Design review of the part built by this model. Coordinates are the model's own, in mm. Face numbers are marked on the shaded views. Give positions to 0.01 mm unless a question says otherwise; leave off trailing zeros. Order: outer loops, then holes, each group sorted by start corner. A loop starts at its lowest first (then second) coordinate and runs counter-clockwise, first axis right, second up. Notation, with made-up numbers: (43.25, -39.75) -> (57.25, -39.75) arc R25 cw to (57.25, -12.75) -> close; hole circle Ø1 at (-4.5, 53). An arc over 180 degrees is marked (long way). Answer in a Markdown table with one row per item. Add a question column.
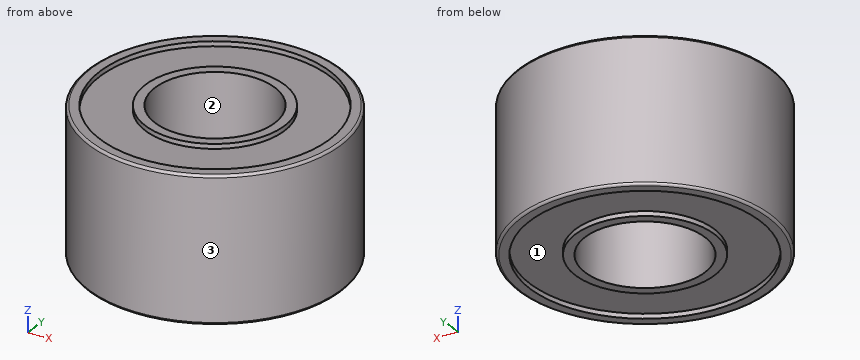
```python
from build123d import *

# Parameters (mm, degrees)
SKETCH1_R           = 10.55
SKETCH1_R_2         = 5
BOSS_EXTRUDE1_DEPTH = 6
FILLET1_R           = 0.2
SKETCH3_R           = 9.602296017
SKETCH3_R_2         = 5.812916565
CUT_EXTRUDE1_DEPTH  = 0.4


with BuildPart() as part:
    # Sketch1 → Boss-Extrude1 (new, symmetric)
    with BuildSketch(Plane.XY):
        Circle(SKETCH1_R)
        Circle(SKETCH1_R_2, mode=Mode.SUBTRACT)
    extrude(amount=BOSS_EXTRUDE1_DEPTH, both=True)

    # Fillet1
    fillet1_edges = [part.edges().sort_by_distance(p)[0] for p in [
        (-10.55, 0, -6),
        (-10.55, 0, 6),
    ]]
    fillet(fillet1_edges, radius=FILLET1_R)

    # Sketch3 → Cut-Extrude1 (cut)
    with BuildSketch(Plane.XY.offset(6)):
        Circle(SKETCH3_R)
        Circle(SKETCH3_R_2, mode=Mode.SUBTRACT)
    cut_extrude1 = extrude(amount=-CUT_EXTRUDE1_DEPTH, mode=Mode.SUBTRACT)

    # Mirror1: Cut-Extrude1 across plane
    add(cut_extrude1.mirror(Plane.XY), mode=Mode.SUBTRACT)


solid = part.part
```
1) Clearance check with flat-ended pins moving along their axes: P1, Ø1.5, axis at y = -1, z = -1, coming from the +X side; P2, Ø3, axis at x = -7, z = -2.5, coming from the -Y side; P3, Ø2, axis at x = 5.5, z = -2, coming from the +Y side. State where each tip first meets the part, or that it passes through.
2) Add section A-A, the plane y = 0. Write out the cut boundary in (x, z).
3) Add section C-C, the plane z = -4.5. Write out the cut boundary in (x, y).
4) Mouldability with a two-part tool opening along X and no side actions: class the marked faces 1, 2 and 3 as +X half, -X half, draft (parallel to the pull), parting line (faces both ways), or undercut.
5) For L1, parallel to Y at x = 0, z = 5.8; L2, parallel to Y at x = 0, z = 0; L3, parallel to Z at x = -1, y = 6.25, list the stretches that pass through material, from the lowest coordinate up.
Verdict:
| question | item | result |
|---|---|---|
| 1 | P1 | stops at x = 10.55 |
| 1 | P2 | stops at y = -9 |
| 1 | P3 | stops at y = 9.54 |
| 2 | outline | (-10.55, -5.8) arc R0.2 ccw to (-10.35, -6) -> (-9.6, -6) -> (-9.6, -5.6) -> (-5.81, -5.6) -> (-5.81, -6) -> (-5, -6) -> (-5, 6) -> (-5.81, 6) -> (-5.81, 5.6) -> (-9.6, 5.6) -> (-9.6, 6) -> (-10.35, 6) arc R0.2 ccw to (-10.55, 5.8) -> close; (5, -6) -> (5.81, -6) -> (5.81, -5.6) -> (9.6, -5.6) -> (9.6, -6) -> (10.35, -6) arc R0.2 ccw to (10.55, -5.8) -> (10.55, 5.8) arc R0.2 ccw to (10.35, 6) -> (9.6, 6) -> (9.6, 5.6) -> (5.81, 5.6) -> (5.81, 6) -> (5, 6) -> close |
| 3 | outline | circle Ø21.1 at (0, 0); hole circle Ø10 at (0, 0) |
| 4 | face 1 | undercut |
| 4 | face 2 | undercut |
| 4 | face 3 | parting line |
| 5 | L1 | y = -10.55 to -9.6, -5.81 to -5, 5 to 5.81, 9.6 to 10.55 |
| 5 | L2 | y = -10.55 to -5, 5 to 10.55 |
| 5 | L3 | z = -5.6 to 5.6 |
